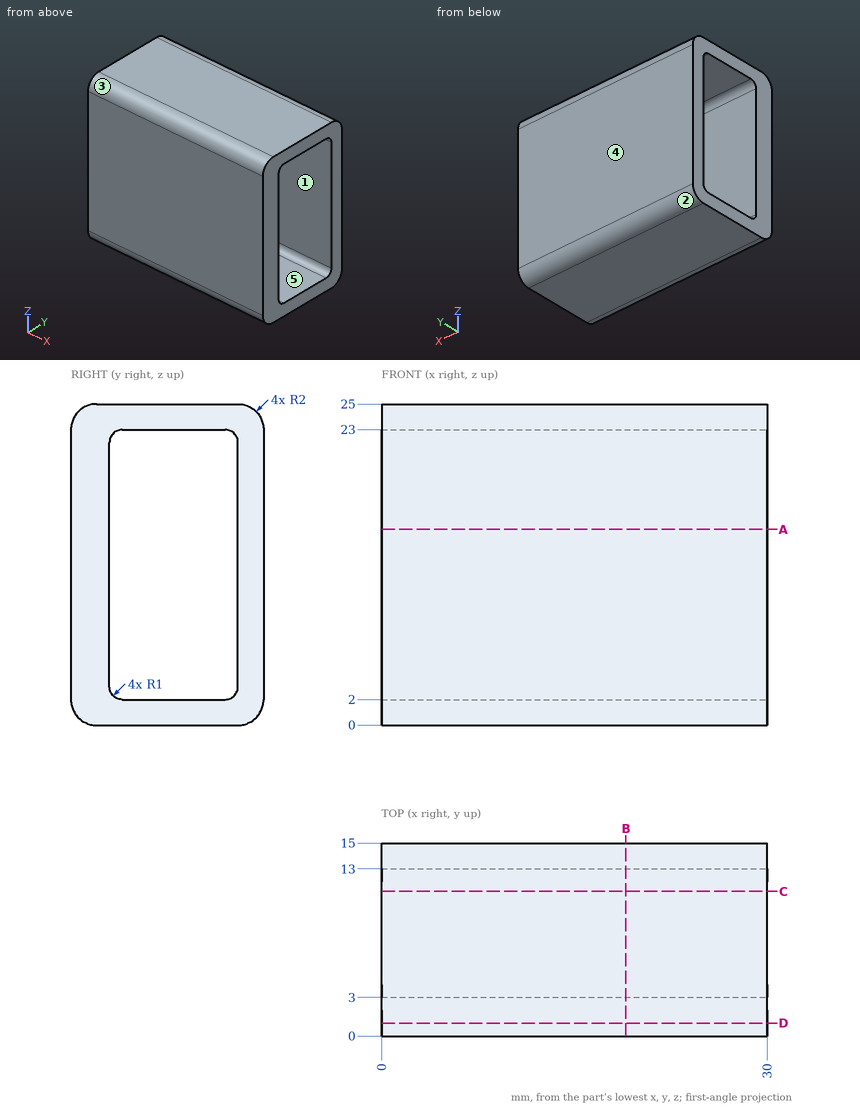
Source: three-view drawing plus pictorial views. Frame: mm from the lowest corner of the part. A direction names the side the tool comes from. Round coordinates to 2 decimals unless told otherwise and drop trailing zeros. Order: outer loops, then holes, each group sorted by start corner. A loop starts at its lowest first (then second) coordinate and runs counter-clockwise, first axis right, second up. Notation, with made-up numbers: (28.5, -22.75) -> (87.5, -22.75) arc R29 cw to (87.5, 0.25) -> close; hole circle Ø6 at (25.25, -7.5). An arc over 180 degrees is marked (long way). Use CSV: the item, a comma, the result in double quotes. Start each with the question number.
1) Section D-D (y = 1). Return the cut outline in (x, z).
2) Material intervals for line 1 along Z through (x, y) = (13.5, 8.25); line 2 along Y through (x, z) = (16.25, 19.5); line 3 along Y through (x, z) = (11.5, 2.5), sorted ascending. Write a range as from..to.
3) Section A-A (z = 15.25). Return the cut outline in (x, y), and give its area (3 significant figures).
4) Section B-B (x = 19). Return the cut outline in (y, z), and give its area (3 significant figures).
5) Section C-C (y = 11.25). Return the cut outline in (x, z).
6) Set-up query: the marked faces 1 and 2. Return all of +Z, -Z, +X, -X, +Y, -Y with unobstructed straight access to the full face (end or side cutting, diameter ignored); none if empty.
7) Draft query along Y for the marked faces 3, 4 and 5. Return one class per face: +Y half, -Y half, draft (parallel to the pull), parting line (faces both ways), or undercut.
Returned:
1,outline,"(0, 0.27) -> (30, 0.27) -> (30, 24.73) -> (0, 24.73) -> close"
2,line 1,"z = 0..2, 23..25"
2,line 2,"y = 0..3, 13..15"
2,line 3,"y = 0..3.13, 12.87..15"
3,outline,"(0, 0) -> (30, 0) -> (30, 3) -> (0, 3) -> close; (0, 13) -> (30, 13) -> (30, 15) -> (0, 15) -> close"
3,area,"150 mm²"
4,outline,"(0, 2) arc R2 ccw to (2, 0) -> (13, 0) arc R2 ccw to (15, 2) -> (15, 23) arc R2 ccw to (13, 25) -> (2, 25) arc R2 ccw to (0, 23) -> close; hole (3, 3) arc R1 ccw to (4, 2) -> (12, 2) arc R1 ccw to (13, 3) -> (13, 22) arc R1 ccw to (12, 23) -> (4, 23) arc R1 ccw to (3, 22) -> close"
4,area,"162 mm²"
5,outline,"(0, 0) -> (30, 0) -> (30, 2) -> (0, 2) -> close; (0, 23) -> (30, 23) -> (30, 25) -> (0, 25) -> close"
6,face 1,"+X, -X"
6,face 2,"-Z, +X, -X, +Y"
7,face 3,"-Y half"
7,face 4,"+Y half"
7,face 5,"undercut"
